```python
from build123d import *

# Parameters (mm, degrees)
BOSS_EXTRUDE2_DEPTH = 3.175
BOSS_EXTRUDE3_DEPTH = 3.175
SKETCH11_W          = 113.03
SKETCH11_H          = 79.94142
BOSS_EXTRUDE8_DEPTH = 3.175
SKETCH12_W          = 70.49262
SKETCH12_H          = 3.175
BOSS_EXTRUDE9_DEPTH = 3.175
SKETCH15_R          = 4.064
CUT_EXTRUDE1_DEPTH  = 371.49176257
SKETCH16_R          = 4.064
CUT_EXTRUDE2_DEPTH  = 371.49176257


with BuildPart() as part:
    # Sketch1 → Boss-Extrude2 (new body)
    with BuildSketch(Plane.XY):
        Polygon((129.013076168, 254.245404572), (-18.685383832, 254.245404572), (-18.685383832, 157.666984572), (92.088461168, 157.666984572), (92.088461168, 154.491984572), (-18.685383832, 154.491984572), (-18.685383832, 57.913564572), (92.088461168, 57.913564572), (92.088461168, 54.738564572), (-18.685383832, 54.738564572), (-18.685383832, -41.839855428), (92.088461168, -41.839855428), (92.088461168, -45.014855428), (-18.685383832, -45.014855428), (-18.685383832, -141.593275428), (92.088461168, -141.593275428), (92.088461168, -144.768275428), (-18.685383832, -144.768275428), (-18.685383832, -241.346695428), (129.013076168, -241.346695428), align=None)
    extrude(amount=BOSS_EXTRUDE2_DEPTH)

    # Sketch4 → Boss-Extrude3 (add, through all)
    with BuildSketch(Plane.XY.offset(3.175)):
        Polygon((129.013076168, 254.245404572), (129.013076168, -241.346695428), (153.407236168, -241.346695428), (153.407236168, -227.262720585), (153.407236168, 240.16142973), (153.407236168, 254.245404572), align=None)
    extrude(amount=-BOSS_EXTRUDE3_DEPTH)

    # Sketch11 → Boss-Extrude8 (add, through all)
    with BuildSketch(Plane.XY.offset(3.175)):
        with Locations((209.922236168, 94.709274572)):
            Rectangle(SKETCH11_W, SKETCH11_H)
    extrude(amount=-BOSS_EXTRUDE8_DEPTH)

    # Sketch12 → Boss-Extrude9 (add, through all)
    with BuildSketch(Plane(origin=(0, 0, 0), x_dir=(-1, 0, 0), z_dir=(0, 0, -1))):
        with Locations((-16.560926168, 255.832904572)):
            Rectangle(SKETCH12_W, SKETCH12_H)
        with Locations((-16.560926168, -242.934195428)):
            Rectangle(SKETCH12_W, SKETCH12_H)
    extrude(amount=-BOSS_EXTRUDE9_DEPTH)

    # Sketch15 → Cut-Extrude1 (cut, through all)
    with BuildSketch(Plane.XY.offset(3.175)):
        with Locations((143.247236168, 231.313297791)):
            Circle(SKETCH15_R)
        with Locations((143.247236168, 164.651984572)):
            Circle(SKETCH15_R)
        with Locations((255.799716168, 113.343984572)):
            Circle(SKETCH15_R)
        with Locations((255.799716168, 74.495671354)):
            Circle(SKETCH15_R)
        with Locations((143.247236168, 29.338564572)):
            Circle(SKETCH15_R)
        with Locations((143.247236168, -32.334232694)):
            Circle(SKETCH15_R)
        with Locations((143.247236168, -94.538012037)):
            Circle(SKETCH15_R)
        with Locations((143.247236168, -156.74179138)):
            Circle(SKETCH15_R)
        with Locations((143.247236168, -218.414588646)):
            Circle(SKETCH15_R)
    extrude(amount=-CUT_EXTRUDE1_DEPTH, mode=Mode.SUBTRACT)

    # Sketch16 → Cut-Extrude2 (cut, through all)
    with BuildSketch(Plane.XY.offset(3.175)):
        with Locations((138.792076168, 121.451235566)):
            Circle(SKETCH16_R)
        with Locations((138.792076168, 82.140925566)):
            Circle(SKETCH16_R)
    extrude(amount=-CUT_EXTRUDE2_DEPTH, mode=Mode.SUBTRACT)


solid = part.part
```
Could you check a few things on this model? Use its own coordinates, in mm. Give positions to 0.01 mm unless a question says otherwise; leave off trailing zeros. Write each loop counter-clockwise with the first axis right and the second up, starting at its lowest first coordinate (ties: lowest second). Pieces come first, ordered by that corner, then holes. Notation, with made-up numbers: (-20, -20.75) - (-1, -20.75) arc R23 ccw to (-1, 9.25) - close; hole circle Ø11 at (8, 48). An arc over 180 degrees is marked (long way). One line per item, written item: value. Start each with the question number.
Item 1: Imagine slicing it at A-A, the plane x = 12. List the corners of the cut face in (y, z) for me (3 decimals), and give its area (3 significant figures).
Item 2: Imagine slicing it at B-B, the plane x = 65.5. List the corners of the cut face in (y, z) for me (3 decimals), and give its area (3 significant figures).
Item 3: Please list where these lines run through material, in increasing order: line 1 (Y direction, x = 91, z = 1.7); line 2 (Y direction, x = 40.5, z = 2.65); line 3 (Y direction, x = 249, z = 1.25). Write a range as from..to.
Item 4: Imagine slicing it at D-D, the plane z = 0.5. Give the number of separate pieces and of enclosed holes in the cut face, and give its area (3 significant figures).
Item 5: I'm going to push flat-ended pins straight in: pin 1 (1 mm diameter, centred on y = 57, z = 2.5, fed in from -X); pin 2 (1.5 mm diameter, centred on x = 54, z = 1, fed in from -Y); pin 3 (1 mm diameter, centred on y = -242.5, z = 1, fed in from +X). Where does each tip first touch, or does it pass through?
Item 6: Imagine slicing it at C-C, the plane x = 223.5. List the corners of the cut face in (y, z) for me (3 decimals), and give its area (3 significant figures).
Geometry says:
1. outline: (-244.522, 0) - (-144.768, 0) - (-144.768, 3.175) - (-244.522, 3.175) - close; (-141.593, 0) - (-45.015, 0) - (-45.015, 3.175) - (-141.593, 3.175) - close; (-41.84, 0) - (54.739, 0) - (54.739, 3.175) - (-41.84, 3.175) - close; (57.914, 0) - (154.492, 0) - (154.492, 3.175) - (57.914, 3.175) - close; (157.667, 0) - (257.42, 0) - (257.42, 3.175) - (157.667, 3.175) - close
1. area: 1,550 mm^2
2. outline: (-241.347, 0) - (-144.768, 0) - (-144.768, 3.175) - (-241.347, 3.175) - close; (-141.593, 0) - (-45.015, 0) - (-45.015, 3.175) - (-141.593, 3.175) - close; (-41.84, 0) - (54.739, 0) - (54.739, 3.175) - (-41.84, 3.175) - close; (57.914, 0) - (154.492, 0) - (154.492, 3.175) - (57.914, 3.175) - close; (157.667, 0) - (254.245, 0) - (254.245, 3.175) - (157.667, 3.175) - close
2. area: 1,530 mm^2
3. line 1: -241.35..-144.77, -141.59..-45.01, -41.84..54.74, 57.91..154.49, 157.67..254.25
3. line 2: -244.52..-144.77, -141.59..-45.01, -41.84..54.74, 57.91..154.49, 157.67..257.42
3. line 3: 54.74..134.68
4. separate pieces: 1
4. enclosed holes: 11
4. area: 92,800 mm^2
5. pin 1: x = 92.09
5. pin 2: y = -241.35
5. pin 3: x = 51.81
6. outline: (54.739, 0) - (134.68, 0) - (134.68, 3.175) - (54.739, 3.175) - close
6. area: 254 mm^2
